from build123d import *

# Parameters (mm, degrees)
F0_R         = 10.5
F1_DEPTH     = 25
F2_R         = 10.5
F3_DEPTH     = 2.5
F4_R         = 2.49999
F5_T4_DEPTH  = 20.1544729749
F5_T10_DEPTH = 20.1544729749
F5_T16_DEPTH = 20.1544729749
F5_T23_DEPTH = 20.1544729749
F5_T27_DEPTH = 20.1544729749
F5_T34_DEPTH = 20.1544729749
F5_T38_DEPTH = 20.1544729749
F5_T45_DEPTH = 20.1544729749
F5_T49_DEPTH = 20.1544729749


# Not quite as in the source:
# - a fillet or chamfer that OpenCascade refuses, or shapes differently, is made with other operations: its cross-section is extruded or revolved along the edge and cut away or added
# - a fillet or chamfer is up to 0.001 mm smaller than in the source, because OpenCascade refuses the exact size


with BuildPart() as f1:
    # F0 (on Front) → F1 (new body)
    with BuildSketch(Plane.XZ):
        Circle(F0_R)
        Polygon((0, -8.6666666667), (-7.5055534995, 4.3333333333), (7.5055534995, 4.3333333333), align=None, mode=Mode.SUBTRACT)
    extrude(amount=F1_DEPTH)

    # F2 (on Front) → F3 (join)
    with BuildSketch(Plane.XZ):
        Circle(F2_R)
    extrude(amount=-F3_DEPTH)

    # F4 (radius 2.5 in the source; OpenCascade refuses exactly that, so slightly less here)
    f4_edges = [f1.edges().sort_by_distance(p)[0] for p in [
        (-10.5, 2.5, 0),
    ]]
    fillet(f4_edges, radius=F4_R)

    # F5: chamfer of 1 on 3 edges, made by hand


with BuildPart() as f5_tool2:
    # F5_s3 → F5_t4 (new body)
    with BuildSketch(Plane(origin=(5.0386182437, 0, -8.7271427981), x_dir=(0, 1, 0), z_dir=(-0.5, 0, 0.8660254038))):
        Polygon((-25, 5.3333333333), (-24, 4.3333333333), (-25, 4.3333333333), align=None)
    extrude(amount=F5_T4_DEPTH)

    split(bisect_by=Plane(origin=(3.7527767497, 0, -2.1666666667), x_dir=(0, 1, 0), z_dir=(-0.8660254038, 0, 0.5)), keep=Keep.TOP)

    split(bisect_by=Plane.XY.offset(4.3333333333), keep=Keep.BOTTOM)


with BuildPart() as f1_1:
    add(f1.part)

    # F5_t1: cut F5_tool2
    add(f5_tool2.part, mode=Mode.SUBTRACT)


with BuildPart() as f5_tool8:
    # F5_s9 → F5_t10 (new body)
    with BuildSketch(Plane.YZ.offset(-10.0772364874)):
        Polygon((-25, 5.3333333333), (-24, 4.3333333333), (-25, 4.3333333333), align=None)
    extrude(amount=F5_T10_DEPTH)

    split(bisect_by=Plane(origin=(3.7527767497, 0, -2.1666666667), x_dir=(0, 1, 0), z_dir=(-0.8660254038, 0, 0.5)), keep=Keep.TOP)

    split(bisect_by=Plane(origin=(-3.7527767497, 0, -2.1666666667), x_dir=(0, 1, 0), z_dir=(0.8660254038, 0, 0.5)), keep=Keep.TOP)


with BuildPart() as f1_2:
    add(f1_1.part)

    # F5_t7: cut F5_tool8
    add(f5_tool8.part, mode=Mode.SUBTRACT)


with BuildPart() as f5_tool14:
    # F5_s15 → F5_t16 (new body)
    with BuildSketch(Plane(origin=(5.0386182437, 0, 8.7271427981), x_dir=(0, 1, 0), z_dir=(-0.5, 0, -0.8660254038))):
        Polygon((-25, 5.3333333333), (-24, 4.3333333333), (-25, 4.3333333333), align=None)
    extrude(amount=F5_T16_DEPTH)

    split(bisect_by=Plane.XY.offset(4.3333333333), keep=Keep.BOTTOM)

    split(bisect_by=Plane(origin=(-3.7527767497, 0, -2.1666666667), x_dir=(0, 1, 0), z_dir=(0.8660254038, 0, 0.5)), keep=Keep.TOP)


with BuildPart() as f1_3:
    add(f1_2.part)

    # F5_t13: cut F5_tool14
    add(f5_tool14.part, mode=Mode.SUBTRACT)


with BuildPart() as f5_tool21:
    # F5_s22 → F5_t23 (new body)
    with BuildSketch(Plane(origin=(5.0386182437, 0, 8.7271427981), x_dir=(0, 1, 0), z_dir=(-0.5, 0, -0.8660254038))):
        Polygon((-25, 5.3333333333), (-24, 4.3333333333), (-25, 4.3333333333), align=None)
    extrude(amount=F5_T23_DEPTH)

    split(bisect_by=Plane(origin=(-3.7527767497, 0, -2.1666666667), x_dir=(0, 1, 0), z_dir=(-0.8660254038, 0, -0.5)), keep=Keep.TOP)


with BuildPart() as f5_tool25:
    # F5_s26 → F5_t27 (new body)
    with BuildSketch(Plane(origin=(5.0386182437, 0, -8.7271427981), x_dir=(0, 1, 0), z_dir=(-0.5, 0, 0.8660254038))):
        Polygon((-25, 5.3333333333), (-24, 4.3333333333), (-25, 4.3333333333), align=None)
    extrude(amount=F5_T27_DEPTH)

    split(bisect_by=Plane(origin=(3.7527767497, 0, -2.1666666667), x_dir=(0, 1, 0), z_dir=(0.8660254038, 0, -0.5)), keep=Keep.TOP)


with BuildPart() as f5_tool21_1:
    add(f5_tool21.part)

    # F5_t29: intersect F5_tool25
    add(f5_tool25.part, mode=Mode.INTERSECT)


with BuildPart() as f1_4:
    add(f1_3.part)

    # F5_t19: cut F5_tool21
    add(f5_tool21_1.part, mode=Mode.SUBTRACT)


with BuildPart() as f5_tool32:
    # F5_s33 → F5_t34 (new body)
    with BuildSketch(Plane(origin=(5.0386182437, 0, -8.7271427981), x_dir=(0, 1, 0), z_dir=(-0.5, 0, 0.8660254038))):
        Polygon((-25, 5.3333333333), (-24, 4.3333333333), (-25, 4.3333333333), align=None)
    extrude(amount=F5_T34_DEPTH)

    split(bisect_by=Plane.XY.offset(4.3333333333), keep=Keep.TOP)


with BuildPart() as f5_tool36:
    # F5_s37 → F5_t38 (new body)
    with BuildSketch(Plane.YZ.offset(-10.0772364874)):
        Polygon((-25, 5.3333333333), (-24, 4.3333333333), (-25, 4.3333333333), align=None)
    extrude(amount=F5_T38_DEPTH)

    split(bisect_by=Plane(origin=(-3.7527767497, 0, -2.1666666667), x_dir=(0, 1, 0), z_dir=(-0.8660254038, 0, -0.5)), keep=Keep.TOP)


with BuildPart() as f5_tool32_1:
    add(f5_tool32.part)

    # F5_t40: intersect F5_tool36
    add(f5_tool36.part, mode=Mode.INTERSECT)


with BuildPart() as f1_5:
    add(f1_4.part)

    # F5_t30: cut F5_tool32
    add(f5_tool32_1.part, mode=Mode.SUBTRACT)


with BuildPart() as f5_tool43:
    # F5_s44 → F5_t45 (new body)
    with BuildSketch(Plane(origin=(5.0386182437, 0, 8.7271427981), x_dir=(0, 1, 0), z_dir=(-0.5, 0, -0.8660254038))):
        Polygon((-25, 5.3333333333), (-24, 4.3333333333), (-25, 4.3333333333), align=None)
    extrude(amount=F5_T45_DEPTH)

    split(bisect_by=Plane.XY.offset(4.3333333333), keep=Keep.TOP)


with BuildPart() as f5_tool47:
    # F5_s48 → F5_t49 (new body)
    with BuildSketch(Plane.YZ.offset(-10.0772364874)):
        Polygon((-25, 5.3333333333), (-24, 4.3333333333), (-25, 4.3333333333), align=None)
    extrude(amount=F5_T49_DEPTH)

    split(bisect_by=Plane(origin=(3.7527767497, 0, -2.1666666667), x_dir=(0, 1, 0), z_dir=(0.8660254038, 0, -0.5)), keep=Keep.TOP)


with BuildPart() as f5_tool43_1:
    add(f5_tool43.part)

    # F5_t51: intersect F5_tool47
    add(f5_tool47.part, mode=Mode.INTERSECT)


with BuildPart() as f1_6:
    add(f1_5.part)

    # F5_t41: cut F5_tool43
    add(f5_tool43_1.part, mode=Mode.SUBTRACT)


solid = f1_6.part
For this review, take the finished solid that the model builds, in its own axes (mm). A direction names the side the tool comes from. Give positions to 0.01 mm unless a question says otherwise; leave off trailing zeros. Loops run counter-clockwise (first coordinate to the right, second up) from the corner with the lowest first, then second, coordinate; pieces in that order, holes last.
Item 1: Tool access review of faces 4 (the flat face through (0, -12, 4.333)), 5 (the flat face through (6, -25, -4)): name each direction out of +Z, -Z, +X, -X, +Y, -Y from which nothing blocks a thin tool from reaching the whole face with its end or side.
Item 2: For line 1 along Y through (x, z) = (-4, 0); line 2 along X through (y, z) = (-22.25, 3.25); line 3 along Z through (x, y) = (2.5, -5.75), list the stretches that pass through material, from the lowest coordinate up.
Item 3: Take a section at B-B, the plane z = 0. State the section outline as (x, y) points, and give its area (3 significant figures).
Item 4: Draft analysis for pull direction X (two halves, no side actions). For faces 1 (the flat face through (0, -25, 7)), 2 (the flat face through (3.805, -11.832, -2.076)), 3 (the cylindrical face through (10, -12.7, 3.2)), state which applies: +X half, -X half, draft (parallel to the pull), parting line (faces both ways), or undercut.
Item 5: Take a section at A-A, the plane y = -1. State the section outline as (x, z) points.
Item 6: Insertion check: pin 1 (4 mm diameter, centred on y = -11, z = 6, fed in from -X); pin 2 (4.5 mm diameter, centred on x = -2.5, y = -18, fed in from -Z); pin 3 (3 mm diameter, centred on y = -8.5, z = -5, fed in from +X); pin 4 (10.5 mm diameter, centred on x = 0, z = -2.5, fed in from -Y). Each pin has a flat end and moves straight along its axis. Give the tip position at first contact, or say it passes through.
Calculated:
1. face 4: -Y
1. face 5: +Z, -Z, +X, -X, -Y
2. line 1: y = 0 to 2.5
2. line 2: x = -9.98 to -6.88, 6.88 to 9.98
2. line 3: z = -10.2 to -4.34, 4.33 to 10.2
3. outline: (-10.5, -25) - (-6.16, -25) - (-5, -24) - (-5, 0) - (5, 0) - (5, -24) - (6.16, -25) - (10.5, -25) - (10.5, 0) arc R2.5 ccw to (8, 2.5) - (-8, 2.5) arc R2.5 ccw to (-10.5, 0) - close
3. area: 323 mm2
4. face 1: draft
4. face 2: undercut
4. face 3: parting line
5. outline: circle Ø21 at (0, 0); hole (-7.51, 4.33) - (0, -8.67) - (7.51, 4.33) - close
6. pin 1: stops at x = -9.71
6. pin 2: stops at z = -10.5
6. pin 3: stops at x = 9.9
6. pin 4: stops at y = -25
